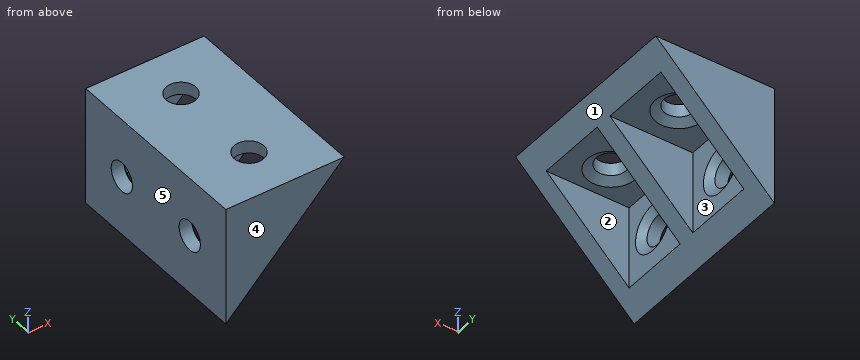
```python
from build123d import *
from OCP.BRepFilletAPI import BRepFilletAPI_MakeChamfer

# Parameters (mm, degrees)
EXTRUDE_1_DEPTH      = 16.5
EXTRUDE_1_DEPTH_BACK = 16.5
EXTRUDE_2_DEPTH      = 3
EXTRUDE_3_DEPTH      = 3
EXTRUDE_4_DEPTH      = 1.5
EXTRUDE_4_DEPTH_BACK = 1.5
SKETCH_5_R           = 2.5
CUT_EXTRUDE_1_DEPTH  = 33.74522866
SKETCH_6_R           = 2.5
CUT_EXTRUDE_2_DEPTH  = 33.74522866
CHAMFER_1_SIZE       = 1.5
CHAMFER_1_SIZE2      = 0.866025404


with BuildPart() as part:
    # Sketch 1 → Extrude 1 (new, two sides: drawn at the far end of the back side and taken through both)
    with BuildSketch(Plane(origin=(0, 0, 0), x_dir=(1, 0, 0), z_dir=(0, 1, 0)).offset(-EXTRUDE_1_DEPTH_BACK)):
        Polygon((0, 0), (0, 20), (3, 17), (3, 3), (17, 3), (20, 0), align=None)
    extrude(amount=EXTRUDE_1_DEPTH + EXTRUDE_1_DEPTH_BACK)

    # Sketch 2 → Extrude 2 (add)
    with BuildSketch(Plane(origin=(0, 16.5, 0), x_dir=(1, 0, 0), z_dir=(0, 1, 0))):
        Polygon((0, 20), (0, 0), (20, 0), align=None)
    extrude(amount=-EXTRUDE_2_DEPTH)

    # Sketch 3 → Extrude 3 (add)
    with BuildSketch(Plane(origin=(0, -16.5, 0), x_dir=(-1, 0, 0), z_dir=(0, -1, 0))):
        Polygon((0, 0), (-20, 0), (0, 20), align=None)
    extrude(amount=-EXTRUDE_3_DEPTH)

    # Sketch 4 → Extrude 4 (add, two sides: drawn at the far end of the back side and taken through both)
    with BuildSketch(Plane(origin=(0, 0, 0), x_dir=(1, 0, 0), z_dir=(0, 1, 0)).offset(-EXTRUDE_4_DEPTH_BACK)):
        Polygon((20, 0), (0, 0), (0, 20), align=None)
    extrude(amount=EXTRUDE_4_DEPTH + EXTRUDE_4_DEPTH_BACK)

    # Sketch 5 → Cut-Extrude 1 (cut, through all)
    with BuildSketch(Plane.XY):
        with Locations((10, 8)):
            Circle(SKETCH_5_R)
        with Locations(Location((10, -8, 0), (0, 0, 180))):
            Circle(SKETCH_5_R)
    extrude(amount=-CUT_EXTRUDE_1_DEPTH, mode=Mode.SUBTRACT)

    # Sketch 6 → Cut-Extrude 2 (cut, through all)
    with BuildSketch(Plane.ZY):
        with Locations((-10, 8)):
            Circle(SKETCH_6_R)
        with Locations(Location((-10, -8, 0), (0, 0, 180))):
            Circle(SKETCH_6_R)
    extrude(amount=-CUT_EXTRUDE_2_DEPTH, mode=Mode.SUBTRACT)

    # Chamfer 1: one chamfer whose edges measure the first distance from different faces: ONE call of the kernel's chamfer builder (chamfer() names one face for all edges)
    chamfer_1_edges_1 = [part.edges().sort_by_distance(p)[0] for p in [
        (12.5, -8, -3),
    ]]
    chamfer_1_side_1 = [part.faces().sort_by_distance(p)[0] for p in [
        (3.184390889, -7.5, -3),
    ]]
    chamfer_1_edges_2 = [part.edges().sort_by_distance(p)[0] for p in [
        (3, 8, -12.5),
    ]]
    chamfer_1_side_2 = [part.faces().sort_by_distance(p)[0] for p in [
        (3, 7.5, -16.815609111),
    ]]
    chamfer_1_edges_3 = [part.edges().sort_by_distance(p)[0] for p in [
        (3, -8, -7.5),
    ]]
    chamfer_1_side_3 = [part.faces().sort_by_distance(p)[0] for p in [
        (3, -7.5, -16.815609111),
    ]]
    chamfer_1_edges_4 = [part.edges().sort_by_distance(p)[0] for p in [
        (7.5, 8, -3),
    ]]
    chamfer_1_side_4 = [part.faces().sort_by_distance(p)[0] for p in [
        (3.184390889, 7.5, -3),
    ]]
    chamfer_1 = BRepFilletAPI_MakeChamfer(part.part.solid().wrapped)
    for e in chamfer_1_edges_1:
        chamfer_1.Add(CHAMFER_1_SIZE, CHAMFER_1_SIZE2, e.wrapped, chamfer_1_side_1[0].wrapped)  # the first distance lies on this face
    for e in chamfer_1_edges_2:
        chamfer_1.Add(CHAMFER_1_SIZE, CHAMFER_1_SIZE2, e.wrapped, chamfer_1_side_2[0].wrapped)  # the first distance lies on this face
    for e in chamfer_1_edges_3:
        chamfer_1.Add(CHAMFER_1_SIZE, CHAMFER_1_SIZE2, e.wrapped, chamfer_1_side_3[0].wrapped)  # the first distance lies on this face
    for e in chamfer_1_edges_4:
        chamfer_1.Add(CHAMFER_1_SIZE, CHAMFER_1_SIZE2, e.wrapped, chamfer_1_side_4[0].wrapped)  # the first distance lies on this face
    add(Compound.cast(chamfer_1.Shape()), mode=Mode.REPLACE)


solid = part.part
```
The listing builds one solid part. Answer for the finished solid, in the listing's coordinates (mm). Face numbers are marked on the shaded views. A direction names the side the tool comes from. Give positions to 0.01 mm unless a question says otherwise; leave off trailing zeros. Loops run counter-clockwise (first coordinate to the right, second up) from the corner with the lowest first, then second, coordinate; pieces in that order, holes last. Notation, with made-up numbers: (88, -4) - (115, -4) arc R18 ccw to (115, 4) - close; hole circle Ø2 at (3, -10). An arc over 180 degrees is marked (long way). Return JSON: item names as keys, results as strings. Group by question number.
1. Find section B-B (x = 10). Write down the section's boundary in (y, z), then the cut area to 3 significant figures.
2. Determine the mould class of the marked faces 3, 4 and 5 for opening direction Y: pulls with the +Y half, pulls with the -Y half, needs draft (parallel to the pull), parting line crosses it, or undercut.
3. Which of the six approach directions +Z, -Z, +X, -X, +Y, -Y give full straight-line access (tool end or side, diameter ignored) to the marked faces 1 and 2?
4. Given pin 1 Ø4 at (x, y) = (8.5, 12) entering from -Z; pin 2 Ø1.5 at (x, y) = (17, -0.5) entering from -Z; pin 3 Ø6 at (y, z) = (-7.5, -10.5) entering from +X, each flat-ended and moving along its own axis, determine where each tip first touches the part or whether it passes through.
5. Find section C-C (y = -8). Write down the section's boundary in (x, z), then the cut area to 3 significant figures.
6. Find section A-A (z = -10). Write down the section's boundary in (x, y), then the cut area to 3 significant figures.
7. Straight lines are drawn through the part: line 1 (Y direction, x = 10, z = -0.7); line 2 (Y direction, x = 11.25, z = -4); line 3 (Z direction, x = 13.25, y = 4.5). For each, find the intervals that lie inside material, in ascending order. Write a range as [from, to].
8. Find section D-D (z = -1.25). Write down the section's boundary in (x, y).
Verdict:
{
 "1": {"outline": "(-16.5, -10) - (-13.5, -10) - (-13.5, -3) - (-12, -3) - (-10.5, -2.13) - (-10.5, 0) - (-16.5, 0) - close; (-5.5, -2.13) - (-4, -3) - (-1.5, -3) - (-1.5, -10) - (1.5, -10) - (1.5, -3) - (4, -3) - (5.5, -2.13) - (5.5, 0) - (-5.5, 0) - close; (10.5, -2.13) - (12, -3) - (13.5, -3) - (13.5, -10) - (16.5, -10) - (16.5, 0) - (10.5, 0) - close", "area": "129 mm^2"},
 "2": {"face 3": "undercut", "face 4": "pulls with the -Y half", "face 5": "needs draft"},
 "3": {"face 1": "-Z, +X, +Y, -Y", "face 2": "-Z, +X"},
 "4": {"pin 1": "stops at z = -12.82", "pin 2": "stops at z = -3.75", "pin 3": "stops at x = 2.83"},
 "5": {"outline": "(0, -20) - (3, -17) - (3, -14) - (2.13, -12.5) - (0, -12.5) - close; (0, -7.5) - (2.13, -7.5) - (3, -6) - (3, -3) - (6, -3) - (7.5, -2.13) - (7.5, 0) - (0, 0) - close; (12.5, -2.13) - (14, -3) - (17, -3) - (20, 0) - (12.5, 0) - close", "area": "69.4 mm^2"},
 "6": {"outline": "(0, -16.5) - (10, -16.5) - (10, -13.5) - (3, -13.5) - (3, -12) - (2.13, -10.5) - (0, -10.5) - close; (0, -5.5) - (2.13, -5.5) - (3, -4) - (3, -1.5) - (10, -1.5) - (10, 1.5) - (3, 1.5) - (3, 4) - (2.13, 5.5) - (0, 5.5) - close; (0, 10.5) - (2.13, 10.5) - (3, 12) - (3, 13.5) - (10, 13.5) - (10, 16.5) - (0, 16.5) - close", "area": "129 mm^2"},
 "7": {"line 1": "y = [-16.5, -10.5], [-5.5, 5.5], [10.5, 16.5]", "line 2": "y = [-16.5, -13.5], [-1.5, 1.5], [13.5, 16.5]", "line 3": "z = [-3, 0]"},
 "8": {"outline": "(0, -16.5) - (18.75, -16.5) - (18.75, 16.5) - (0, 16.5) - close; hole circle Ø5 at (10, -8); hole circle Ø5 at (10, 8)"}
}
